from build123d import *

# Parameters (mm, degrees)
F0_R     = 12
F1_DEPTH = 50
F0_R_2   = 47.5
F2_DEPTH = 3
F0_R_3   = 70
F3_DEPTH = 260


with BuildPart() as f1:
    # F0 (on Front) → F1 (new body)
    with BuildSketch(Plane.XZ):
        Circle(F0_R)
    extrude(amount=F1_DEPTH)

    # F0 (on Front) → F2 (join)
    with BuildSketch(Plane.XZ):
        Circle(F0_R_2)
        Circle(F0_R, mode=Mode.SUBTRACT)
    extrude(amount=F2_DEPTH)

    # F0 (on Front) → F3 (join)
    with BuildSketch(Plane.XZ):
        Circle(F0_R_3)
        Circle(F0_R_2, mode=Mode.SUBTRACT)
        Circle(F0_R_2)
        Circle(F0_R, mode=Mode.SUBTRACT)
        Circle(F0_R)
    extrude(amount=-F3_DEPTH)


solid = f1.part
The listing builds one solid part. Answer for the finished solid, in the listing's coordinates (mm). A direction names the side the tool comes from. Round coordinates to 2 decimals unless told otherwise and drop trailing zeros. Loops run counter-clockwise (first coordinate to the right, second up) from the corner with the lowest first, then second, coordinate; pieces in that order, holes last. Notation, with made-up numbers: M 61.25,10.5 L 117.25,10.5 A25 cw 117.25,47.5 Z; hole C 9.25,-26.75 d3. An arc over 180 degrees is marked long. Write each question's results on one line, items separated by ' | '. Start each with the question number.
1) Straight lines are drawn through the part: probe 1 along Y at (x, z) = (43.5, -51); probe 2 along Y at (x, z) = (-26.5, -0.5); probe 3 along X at (y, z) = (186.5, 1). For each, find the intervals that lie inside material, in ascending order.
2) Find section C-C on y = 43. Write down the section's boundary in (x, z), plus the area to 3 significant figures.
3) Find section B-B on z = 26.5. Write down the section's boundary in (x, y), plus the area to 3 significant figures.
4) Find section D-D on z = 0. Write down the section's boundary in (x, y), plus the area to 3 significant figures.
5) Which of the six approach directions +Z, -Z, +X, -X, +Y, -Y give full straight-line access (tool end or side, diameter ignored) to faces 1 (the cylindrical face through (-55.55, 128.18, -42.594)), 2 (the cylindrical face through (-10.3, -1.48, -46.37))?
6) Find section A-A on x = 0. Write down the section's boundary in (y, z), plus the area to 3 significant figures.
7) Each of these flat-tipped pins is pushed along its axis until it touches: pin 1 (1 mm diameter, centred on x = 22, y = 141, fed in from -Z); pin 2 (3 mm diameter, centred on x = 20, y = 155, fed in from -Z); pin 3 (4 mm diameter, centred on x = -33, z = -8.5, fed in from -Y). Where does it stop, or does it pass through?
Final values:
1) probe 1: 0 to 260 | probe 2: -3 to 260 | probe 3: -69.99 to 69.99
2) outline: C 0,0 d140 | area: 15,400 mm²
3) outline: M -64.79,0 L -39.42,0 L -39.42,-3 L 39.42,-3 L 39.42,0 L 64.79,0 L 64.79,260 L -64.79,260 Z | area: 33,900 mm²
4) outline: M -70,0 L -47.5,0 L -47.5,-3 L -12,-3 L -12,-50 L 12,-50 L 12,-3 L 47.5,-3 L 47.5,0 L 70,0 L 70,260 L -70,260 Z | area: 37,800 mm²
5) face 1: +Y, -Y | face 2: -Y
6) outline: M -50,-12 L -3,-12 L -3,-47.5 L 0,-47.5 L 0,-70 L 260,-70 L 260,70 L 0,70 L 0,47.5 L -3,47.5 L -3,12 L -50,12 Z | area: 37,800 mm²
7) pin 1: z = -66.62 | pin 2: z = -67.51 | pin 3: y = -3
